Source: CAD feature listing. Evaluate the final solid. Frame: model axes, mm. A direction names the side the tool comes from. Give positions to 0.01 mm unless a question says otherwise; leave off trailing zeros. Loops run counter-clockwise (first coordinate to the right, second up) from the corner with the lowest first, then second, coordinate; pieces in that order, holes last. Notation, with made-up numbers: (80.5, -17) - (104.5, -17) arc R12 ccw to (104.5, -12) - close; hole circle Ø10 at (7, 37). An arc over 180 degrees is marked (long way). Put each result on its own line as item: value.
```python
from build123d import *

# Parameters (mm, degrees)
SKETCH_2_W          = 140
SKETCH_2_H          = 140
EXTRUDE_1_DEPTH     = 4
EXTRUDE_1_2_DEPTH   = 100
EXTRUDE_2_DEPTH     = 2
CUT_EXTRUDE_1_DEPTH = 95.5
SKETCH_6_R          = 6.5
CUT_EXTRUDE_2_DEPTH = 5
FILLET_1_R          = 10


with BuildPart() as part:
    # Эскиз2 → Extrude 1 (new body)
    with BuildSketch(Plane(origin=(0, 0, 0), x_dir=(1, 0, 0), z_dir=(0, 1, 0))):
        Rectangle(SKETCH_2_W, SKETCH_2_H)
    extrude(amount=EXTRUDE_1_DEPTH)

    # Эскиз3 → Extrude 1 2 (add)
    with BuildSketch(Plane(origin=(0, 4, 0), x_dir=(1, 0, 0), z_dir=(0, 1, 0))):
        with BuildLine():
            Line((-20.5, -20), (-20.5, 19))
            ThreePointArc((-20.5, 19), (-20.207106781, 19.707106781), (-19.5, 20))
            Line((-19.5, 20), (19.5, 20))
            ThreePointArc((19.5, 20), (20.207106781, 19.707106781), (20.5, 19))
            Line((20.5, 19), (20.5, -20))
            Line((20.5, -20), (24.5, -20))
            Line((24.5, -20), (24.5, 19))
            ThreePointArc((24.5, 19), (23.035533906, 22.535533906), (19.5, 24))
            Line((19.5, 24), (-19.5, 24))
            ThreePointArc((-19.5, 24), (-23.035533906, 22.535533906), (-24.5, 19))
            Line((-24.5, 19), (-24.5, -20))
            Line((-24.5, -20), (-20.5, -20))
        make_face()
    extrude(amount=EXTRUDE_1_2_DEPTH)

    # Эскиз4 → Бобышка-Вытянуть2 (add, symmetric)
    with BuildSketch(Plane(origin=(0, 0, 0), x_dir=(0, 0, -1), z_dir=(1, 0, 0))):
        Polygon((24, 75.01408311), (65, 4), (24, 4), align=None)
    extrude(amount=EXTRUDE_2_DEPTH, both=True)

    # Эскиз5 → Вырез-Вытянуть1 (cut, through all)
    with BuildSketch(Plane(origin=(24.5, 0, 0), x_dir=(0, 0, -1), z_dir=(1, 0, 0))):
        with BuildLine():
            Line((5, 92), (5, 80))
            ThreePointArc((5, 80), (0, 75), (-5, 80))
            Line((-5, 80), (-5, 92))
            ThreePointArc((-5, 92), (0, 97), (5, 92))
        make_face()
        with BuildLine():
            Line((5, 28), (5, 16))
            ThreePointArc((5, 16), (0, 11), (-5, 16))
            Line((-5, 16), (-5, 28))
            ThreePointArc((-5, 28), (0, 33), (5, 28))
        make_face()
    extrude(amount=-CUT_EXTRUDE_1_DEPTH, mode=Mode.SUBTRACT)

    # Эскиз6 → Вырез-Вытянуть2 (cut, through all)
    with BuildSketch(Plane(origin=(0, 4, 0), x_dir=(1, 0, 0), z_dir=(0, 1, 0))):
        with Locations(Location((-55, 55, 0), (0, 0, 270))):  # turned: the seam where the file's is
            Circle(SKETCH_6_R)
        with Locations(Location((-55, -55, 0), (0, 0, 270))):  # turned: the seam where the file's is
            Circle(SKETCH_6_R)
        with Locations(Location((55, 55, 0), (0, 0, 270))):  # turned: the seam where the file's is
            Circle(SKETCH_6_R)
        with Locations(Location((55, -55, 0), (0, 0, 270))):  # turned: the seam where the file's is
            Circle(SKETCH_6_R)
    extrude(amount=-CUT_EXTRUDE_2_DEPTH, mode=Mode.SUBTRACT)

    # Скругление1
    fillet_1_edges = [part.edges().sort_by_distance(p)[0] for p in [
        (70, 2, 70),
        (-70, 2, 70),
        (-70, 2, -70),
        (70, 2, -70),
    ]]
    fillet(fillet_1_edges, radius=FILLET_1_R)


solid = part.part
```
1) Section query B-B, the plane x = -57.5. Output: boundary loops of the cut face in (y, z).
Check result:
outline: (0, -70) - (4, -70) - (4, -61) - (0, -61) - close; (0, -49) - (4, -49) - (4, 49) - (0, 49) - close; (0, 61) - (4, 61) - (4, 70) - (0, 70) - close
2) Section query D-D, the plane x = -13. Output: boundary loops of the cut face in (y, z), plus the area to 3 significant figures.
Check result:
outline: (0, -70) - (4, -70) - (4, -24) - (104, -24) - (104, -20) - (4, -20) - (4, 70) - (0, 70) - close
area: 960 mm²
3) Pin query (flat end, axial travel): P1, Ø10, axis at y = 36, z = 13, coming from the +X side; P2, Ø12.5, axis at y = 40.5, z = -40.5, coming from the -X side; P3, Ø5, axis at x = -15.5, z = 34.5, coming from the +Y side. Return the tip coordinate at first contact, or that it passes through.
Check result:
P1: x = 24.5
P2: x = -2
P3: y = 4
4) Material intervals for line 1 along X through (y, z) = (2.8, -55); line 2 along X through (y, z) = (40, 3); line 3 along Z through (x, y) = (3.5, 68), sorted ascending. Write a range as [from, to].
Check result:
line 1: [-70, -61.5], [-48.5, 48.5], [61.5, 70]
line 2: [-24.5, -20.5], [20.5, 24.5]
line 3: [-24, -20]
5) Section query A-A, the plane z = 55. Output: boundary loops of the cut face in (x, y), plus the area to 3 significant figures.
Check result:
outline: (-70, 0) - (-61.5, 0) - (-61.5, 4) - (-70, 4) - close; (-48.5, 0) - (48.5, 0) - (48.5, 4) - (-48.5, 4) - close; (61.5, 0) - (70, 0) - (70, 4) - (61.5, 4) - close
area: 456 mm²
6) Mould query, pull axis X, two halves, no side actions, for faces 1 (the cylindrical face through (49.233, 2.028, -52.001)), 2 (the cylindrical face through (23.07, 53.3, -22.5)), 3 (the cylindrical face through (23, 97, 0)). Classes: pulls with the +X half, pulls with the -X half, needs draft (parallel to the pull), parting line crosses it, or undercut.
Check result:
face 1: undercut
face 2: pulls with the +X half
face 3: needs draft
7) Section query C-C, the plane y = 23.5. Output: boundary loops of the cut face in (x, z).
Check result:
outline: (-24.5, -19) arc R5 ccw to (-19.5, -24) - (-2, -24) - (-2, -53.74) - (2, -53.74) - (2, -24) - (19.5, -24) arc R5 ccw to (24.5, -19) - (24.5, -5) - (20.5, -5) - (20.5, -19) arc R1 cw to (19.5, -20) - (-19.5, -20) arc R1 cw to (-20.5, -19) - (-20.5, -5) - (-24.5, -5) - close; (-24.5, 5) - (-20.5, 5) - (-20.5, 20) - (-24.5, 20) - close; (20.5, 5) - (24.5, 5) - (24.5, 20) - (20.5, 20) - close
8) Access query for faces 4 (the flat face through (22, 53, 20)), 5 (the flat face through (20.5, 53, 0)), 6 (the cylindrical face through (-23, 53.3, -22.57)), 7 (the cylindrical face through (-22, 33, 0)), 8 (the flat face through (70, 2, 1)). Directions: +Z, -Z, +X, -X, +Y, -Y. A direction counts if a zero-diameter tool reaches every point of the face in a straight line with its end or side. Return the directions, or none.
Check result:
face 4: +Z, +X, -X, +Y
face 5: +Z, +Y
face 6: -Z, -X, +Y
face 7: +X, -X
face 8: +Z, -Z, +X, +Y, -Y
